from build123d import *

# Parameters (mm, degrees)
SKETCH1_W           = 35
SKETCH1_H           = 41
BOSS_EXTRUDE1_DEPTH = 5
SKETCH2_R           = 1.5
CUT_EXTRUDE1_DEPTH  = 5
SKETCH3_W           = 35
SKETCH3_H           = 31
BOSS_EXTRUDE2_DEPTH = 73.1
SKETCH4_W           = 26
SKETCH4_H           = 7
CUT_EXTRUDE2_DEPTH  = 30
SKETCH5_R           = 2.4
CUT_EXTRUDE3_DEPTH  = 8
FILLET1_R           = 5
FILLET2_R           = 5


with BuildPart() as part:
    # Sketch1 → Boss-Extrude1 (new body)
    with BuildSketch(Plane(origin=(0, 0, 0), x_dir=(1, 0, 0), z_dir=(0, 1, 0))):
        with Locations((17.5, 20.5)):
            Rectangle(SKETCH1_W, SKETCH1_H)
    extrude(amount=BOSS_EXTRUDE1_DEPTH)

    # Sketch2 → Cut-Extrude1 (cut)
    with BuildSketch(Plane(origin=(0, 5, 0), x_dir=(1, 0, 0), z_dir=(0, 1, 0))):
        with Locations(Location((7.5, 5, 0), (0, 0, 270))):
            Circle(SKETCH2_R)
        with Locations(Location((27.5, 5, 0), (0, 0, 270))):
            Circle(SKETCH2_R)
    extrude(amount=-CUT_EXTRUDE1_DEPTH, mode=Mode.SUBTRACT)

    # Sketch3 → Boss-Extrude2 (add)
    with BuildSketch(Plane(origin=(0, 5, 0), x_dir=(1, 0, 0), z_dir=(0, 1, 0))):
        with Locations((17.5, 25.5)):
            Rectangle(SKETCH3_W, SKETCH3_H)
    extrude(amount=BOSS_EXTRUDE2_DEPTH)

    # Sketch4 → Cut-Extrude2 (cut)
    with BuildSketch(Plane(origin=(35, 0, 0), x_dir=(0, 0, -1), z_dir=(1, 0, 0))):
        with Locations((28, 66.6)):
            Rectangle(SKETCH4_W, SKETCH4_H)
    extrude(amount=-CUT_EXTRUDE2_DEPTH, mode=Mode.SUBTRACT)

    # Sketch5 → Cut-Extrude3 (cut)
    with BuildSketch(Plane(origin=(0, 78.1, 0), x_dir=(1, 0, 0), z_dir=(0, 1, 0))):
        with Locations(Location((18, 30.202102686, 0), (0, 0, 270))):
            Circle(SKETCH5_R)
    extrude(amount=-CUT_EXTRUDE3_DEPTH, mode=Mode.SUBTRACT)

    # Fillet1
    fillet1_edges = [part.edges().sort_by_distance(p)[0] for p in [
        (0, 78.1, -25.5),
    ]]
    fillet(fillet1_edges, radius=FILLET1_R)

    # Fillet2
    fillet2_edges = [part.edges().sort_by_distance(p)[0] for p in [
        (20, 78.1, -10),
        (0, 39.05, -10),
        (1.464466094, 76.635533906, -10),
    ]]
    fillet(fillet2_edges, radius=FILLET2_R)


solid = part.part
Geometry check sheet. Reference: the model listing, model coordinates, mm. A direction names the side the tool comes from. Give positions to 0.01 mm unless a question says otherwise; leave off trailing zeros. Loops run counter-clockwise (first coordinate to the right, second up) from the corner with the lowest first, then second, coordinate; pieces in that order, holes last.
(1) Section check C-C on y = 67.5. Record the cut outline in (x, z), then the cut area to 3 significant figures.
From the geometry:
outline: (0, -41) - (5, -41) - (5, -15) - (35, -15) - (35, -10) - (5, -10) arc R5 ccw to (0, -15) - close
area: 300 mm2
(2) Section check B-B on x = 18. Record the cut outline in (y, z), then the cut area to 3 significant figures.
From the geometry:
outline: (0, -41) - (63.1, -41) - (63.1, -15) - (70.1, -15) - (70.1, -27.8) - (78.1, -27.8) - (78.1, -15) arc R5 ccw to (73.1, -10) - (5, -10) - (5, 0) - (0, 0) - close; (70.1, -41) - (78.1, -41) - (78.1, -32.6) - (70.1, -32.6) - close
area: 2,250 mm2
(3) Depth check by flat-ended pin: pin 1 Ø3 at (y, z) = (67.5, -25.5) entering from +X; pin 2 Ø4.5 at (x, z) = (18, -30.2) entering from +Y; pin 3 Ø5 at (x, y) = (20, 47) entering from +Z; pin 4 Ø2.5 at (x, z) = (7.5, -5) entering from +Y. Enter the tip coordinate at first touch or a pass-through.
From the geometry:
pin 1: stops at x = 5
pin 2: stops at y = 63.1
pin 3: stops at z = -10
pin 4: passes through
(4) Release check for a two-part mould opening along Y. For faces 5 (the flat face through (5, 67, -28)), 6 (the flat face through (20, 39, -10)), 7 (the flat face through (17, 0, -21)) record: released by +Y, released by -Y, zero draft, split by the parting line, or undercut.
From the geometry:
face 5: undercut
face 6: zero draft
face 7: released by -Y
(5) Thickness scan on L1, parallel to X at y = 2.85, z = -5; L2, parallel to Y at x = 14, z = -20.5; L3, parallel to Z at x = 26, y = 59.5. Record the ranges inside material, lowest first.
From the geometry:
L1: x = 0 to 6, 9 to 26, 29 to 35
L2: y = 0 to 63.1, 70.1 to 78.1
L3: z = -41 to -10
(6) Set-up check for faces 1 (the cylindrical face through (2, 40, -11)), 2 (the cylindrical face through (17.081, 74.156, -27.985)), 3 (the flat face through (20, 63.1, -28)), 4 (the cylindrical face through (1.43, 76.6, -28.18)): record each of +Z, -Z, +X, -X, +Y, -Y from which the full face is reachable in a straight line by a thin tool's end or side.
From the geometry:
face 1: +Z, -X, +Y
face 2: +Y
face 3: -Z, +X
face 4: +Z, -Z, -X, +Y
(7) Section check A-A on z = -5. Record the cut outline in (x, y).
From the geometry:
outline: (0, 0) - (6, 0) - (6, 5) - (0, 5) - close; (9, 0) - (26, 0) - (26, 5) - (9, 5) - close; (29, 0) - (35, 0) - (35, 5) - (29, 5) - close
(8) Section check D-D on z = -21.5. Record the cut outline in (x, y), then the cut area to 3 significant figures.
From the geometry:
outline: (0, 0) - (35, 0) - (35, 63.1) - (5, 63.1) - (5, 70.1) - (35, 70.1) - (35, 78.1) - (5, 78.1) arc R5 ccw to (0, 73.1) - close
area: 2,520 mm2
